```python
from build123d import *

# Parameters (mm, degrees)
BOSS_EXTRUDE2_DEPTH     = 6.35
SKETCH2_W               = 19.05
SKETCH2_H               = 13.716
CUT_EXTRUDE1_DEPTH      = 7.35
SKETCH3_R               = 38.1
CUT_EXTRUDE2_DEPTH      = 7.35
FILLET1_R               = 6.35
SKETCH7_R               = 3.175
CUT_EXTRUDE6_DEPTH      = 103.378
CUT_EXTRUDE6_DEPTH_BACK = 1.0000001
SKETCH8_R               = 1.651
CUT_EXTRUDE7_DEPTH      = 75.692
SKETCH10_R              = 1.651
CUT_EXTRUDE9_DEPTH      = 97.79
SKETCH11_R              = 1.651
CUT_EXTRUDE10_DEPTH     = 150.876
SKETCH12_R              = 6.35
CUT_EXTRUDE11_DEPTH     = 31.242


with BuildPart() as part:
    # Sketch1 → Boss-Extrude2 (new body)
    with BuildSketch(Plane.XY):
        with BuildLine():
            ThreePointArc((-69.525975721, 27.94), (-74.93, 0), (-69.525975721, -27.94))
            ThreePointArc((-69.525975721, -27.94), (0, -74.93), (69.525975721, -27.94))
            ThreePointArc((69.525975721, -27.94), (73.56658977, -14.228906128), (74.93, 0))
            ThreePointArc((74.93, 0), (73.56658977, 14.228906128), (69.525975721, 27.94))
            ThreePointArc((69.525975721, 27.94), (0, 74.93), (-69.525975721, 27.94))
        make_face()
        with BuildLine():
            ThreePointArc((-67.493975721, 26.416), (-67.122001333, 27.314025612), (-66.223975721, 27.686))
            Line((-66.223975721, 27.686), (-56.063975721, 27.686))
            Line((-56.063975721, 27.686), (-56.063975721, -27.686))
            Line((-56.063975721, -27.686), (-66.223975721, -27.686))
            ThreePointArc((-66.223975721, -27.686), (-67.122001333, -27.314025612), (-67.493975721, -26.416))
            Line((-67.493975721, -26.416), (-67.493975721, 26.416))
        make_face(mode=Mode.SUBTRACT)
        with BuildLine():
            ThreePointArc((66.223975721, 27.686), (67.122001333, 27.314025612), (67.493975721, 26.416))
            Line((67.493975721, 26.416), (67.493975721, -26.416))
            ThreePointArc((67.493975721, -26.416), (67.122001333, -27.314025612), (66.223975721, -27.686))
            Line((66.223975721, -27.686), (56.063975721, -27.686))
            Line((56.063975721, -27.686), (56.063975721, 27.686))
            Line((56.063975721, 27.686), (66.223975721, 27.686))
        make_face(mode=Mode.SUBTRACT)
    extrude(amount=BOSS_EXTRUDE2_DEPTH)

    # Sketch2 → Cut-Extrude1 (cut, through all)
    with BuildSketch(Plane.XY.offset(6.35)):
        with Locations((0, 62.23)):
            Rectangle(SKETCH2_W, SKETCH2_H)
    extrude(amount=-CUT_EXTRUDE1_DEPTH, mode=Mode.SUBTRACT)

    # Sketch3 → Cut-Extrude2 (cut, through all)
    with BuildSketch(Plane.XY.offset(6.35)):
        with Locations((0, -86.312058398)):
            Circle(SKETCH3_R)
    extrude(amount=-CUT_EXTRUDE2_DEPTH, mode=Mode.SUBTRACT)

    # Fillet1
    fillet1_edges = [part.edges().sort_by_distance(p)[0] for p in [
        (-33.000960548, -67.271401821, 3.175),
        (33.000960548, -67.271401821, 3.175),
    ]]
    fillet(fillet1_edges, radius=FILLET1_R)

    # Sketch7 → Cut-Extrude6 (cut, two sides)
    with BuildSketch(Plane(origin=(30.092005081, 4.08352975, 6.35), x_dir=(-1, 0, 0), z_dir=(0, 0, -1))) as cut_extrude6_sk:
        with Locations((-13.087994919, 21.31647025)):
            Circle(SKETCH7_R)
        with Locations((73.272005081, 21.31647025)):
            Circle(SKETCH7_R)
        with Locations((30.092005081, 21.31647025)):
            Circle(SKETCH7_R)
        with Locations((73.272005081, -29.48352975)):
            Circle(SKETCH7_R)
        with Locations((30.092005081, -29.48352975)):
            Circle(SKETCH7_R)
        with Locations((-13.087994919, -29.48352975)):
            Circle(SKETCH7_R)
    extrude(amount=CUT_EXTRUDE6_DEPTH, mode=Mode.SUBTRACT)
    extrude(cut_extrude6_sk.sketch, amount=-CUT_EXTRUDE6_DEPTH_BACK, mode=Mode.SUBTRACT)

    # Sketch8 → Cut-Extrude7 (cut)
    with BuildSketch(Plane(origin=(30.092005081, 4.08352975, -35.052), x_dir=(-1, 0, 0), z_dir=(0, 0, -1))):
        with Locations((63.757223581, 17.50647025)):
            Circle(SKETCH8_R)
        with Locations((63.757223581, -25.67352975)):
            Circle(SKETCH8_R)
        with Locations((-3.552776419, -25.67352975)):
            Circle(SKETCH8_R)
        with Locations((-3.552776419, 17.50647025)):
            Circle(SKETCH8_R)
    extrude(amount=-CUT_EXTRUDE7_DEPTH, mode=Mode.SUBTRACT)

    # Sketch10 → Cut-Extrude9 (cut)
    with BuildSketch(Plane(origin=(30.092005081, 4.08352975, -41.275), x_dir=(-1, 0, 0), z_dir=(0, 0, -1))):
        with Locations((4.154396091, -49.728759131)):
            Circle(SKETCH10_R)
        with Locations((56.02961407, -49.728759131)):
            Circle(SKETCH10_R)
        with Locations((4.154396091, 41.38247025)):
            Circle(SKETCH10_R)
        with Locations((56.02961407, 41.38247025)):
            Circle(SKETCH10_R)
    extrude(amount=-CUT_EXTRUDE9_DEPTH, mode=Mode.SUBTRACT)

    # Sketch11 → Cut-Extrude10 (cut)
    with BuildSketch(Plane(origin=(30.092005081, 4.08352975, 6.35), x_dir=(1, 0, 0), z_dir=(0, 0, 1))):
        with Locations((-101.395980802, -12.71952975)):
            Circle(SKETCH11_R)
        with Locations((-101.395980802, 4.55247025)):
            Circle(SKETCH11_R)
        with Locations((41.211970641, -12.71952975)):
            Circle(SKETCH11_R)
        with Locations((41.211970641, 4.55247025)):
            Circle(SKETCH11_R)
    extrude(amount=-CUT_EXTRUDE10_DEPTH, mode=Mode.SUBTRACT)

    # Sketch12 → Cut-Extrude11 (cut)
    with BuildSketch(Plane.XY.offset(6.35)):
        with Locations((0, 25.4)):
            Circle(SKETCH12_R)
        with Locations((-43.18, 25.4)):
            Circle(SKETCH12_R)
        with Locations((-43.18, -25.4)):
            Circle(SKETCH12_R)
        with Locations((0, -25.4)):
            Circle(SKETCH12_R)
        with Locations((43.18, -25.4)):
            Circle(SKETCH12_R)
        with Locations((43.18, 25.4)):
            Circle(SKETCH12_R)
    extrude(amount=-CUT_EXTRUDE11_DEPTH, mode=Mode.SUBTRACT)


solid = part.part
```
The listing builds one solid part. Answer for the finished solid, in the listing's coordinates (mm). Round coordinates to 2 decimals unless told otherwise and drop trailing zeros. Loops run counter-clockwise (first coordinate to the right, second up) from the corner with the lowest first, then second, coordinate; pieces in that order, holes last. Notation, with made-up numbers: (38.25, -24) - (53.25, -24) arc R27 cw to (53.25, 2) - close; hole circle Ø11 at (3.25, 79.5). An arc over 180 degrees is marked (long way). Return JSON: item names as keys, results as strings. Group by question number.
1. The part is cut by section A-A on x = 0. Determine the outline of the cut face in (y, z), then the cut area to 3 significant figures.
2. The part is cut by section B-B on y = -4. Determine the outline of the cut face in (x, z), then the cut area to 3 significant figures.
3. Each of these flat-tipped pins is pushed along its axis until it touches: P1, Ø1, axis at x = 29.5, z = 4.5, coming from the +Y side; P2, Ø1.9, axis at y = 63.5, z = 4, coming from the +X side; P3, Ø1.5, axis at y = -24, z = 5.5, coming from the -X side. Where does it stop, or does it pass through?
4. The part is cut by section C-C on x = -46. Determine the outline of the cut face in (y, z).
5. The mould has two halves that part along Y. Classify faces 1 (the flat face through (-1, 6, 0)), 2 (the cylindrical face through (26.296, 43.854, 3.131)): pulls with the +Y half, pulls with the -Y half, needs draft (parallel to the pull), parting line crosses it, or undercut.
6. The part is cut by section D-D on y = -21.59. State how many separate pieces and enclosed holes the cut face has, then the cut area to 3 significant figures.
7. Consider probe 1 along Y at (x, z) = (-25.5, 6.25); probe 2 along X at (y, z) = (-13, 3.75); probe 3 along X at (y, z) = (12.5, 0.75). Determine where each line is inside the solid, lowest interval first.
Resolved:
{
 "1": {"outline": "(-48.21, 0) - (-31.75, 0) - (-31.75, 6.35) - (-48.21, 6.35) - close; (-19.05, 0) - (19.05, 0) - (19.05, 6.35) - (-19.05, 6.35) - close; (31.75, 0) - (55.37, 0) - (55.37, 6.35) - (31.75, 6.35) - close; (69.09, 0) - (74.93, 0) - (74.93, 6.35) - (69.09, 6.35) - close", "area": "534 mm²"},
 "2": {"outline": "(-74.82, 0) - (-67.49, 0) - (-67.49, 6.35) - (-74.82, 6.35) - close; (-56.06, 0) - (56.06, 0) - (56.06, 6.35) - (-56.06, 6.35) - close; (67.49, 0) - (74.82, 0) - (74.82, 6.35) - (67.49, 6.35) - close", "area": "805 mm²"},
 "3": {"P1": "stops at y = 69.09", "P2": "stops at x = 41.26", "P3": "stops at x = -71.23"},
 "4": {"outline": "(-59.15, 0) - (-31.09, 0) - (-31.09, 6.35) - (-59.15, 6.35) - close; (-19.71, 0) - (19.71, 0) - (19.71, 6.35) - (-19.71, 6.35) - close; (31.09, 0) - (59.15, 0) - (59.15, 6.35) - (31.09, 6.35) - close"},
 "5": {"face 1": "needs draft", "face 2": "undercut"},
 "6": {"separate pieces": "8", "enclosed holes": "0", "area": "531 mm²"},
 "7": {"probe 1": "y = -58 to -47.24, -44.05 to 43.87, 47.06 to 70.46", "probe 2": "x = -73.79 to -67.49, -56.06 to 56.06, 67.49 to 73.79", "probe 3": "x = -73.88 to -67.49, -56.06 to 56.06, 67.49 to 73.88"}
}
